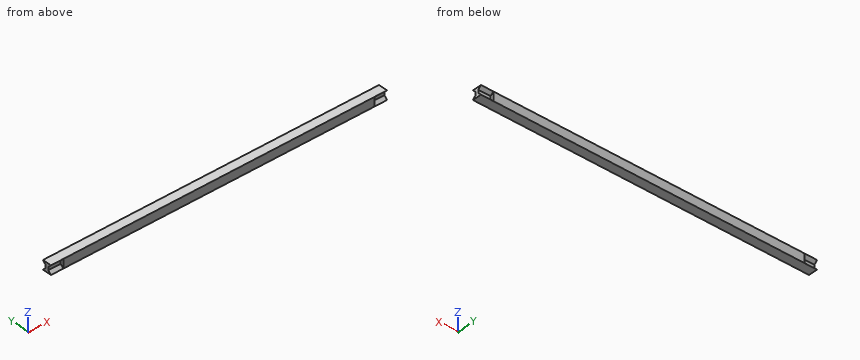
from build123d import *

# Parameters (mm, degrees)
SKICA1_W                = 202
SKICA1_H                = 5.9
P_IDAT_VYSUNUT_M1_DEPTH = 5.9
P_IDAT_VYSUNUT_M2_DEPTH = 8
P_IDAT_VYSUNUT_M3_DEPTH = 8


with BuildPart() as part:
    # Skica1 → Přidat vysunutím1 (new body)
    with BuildSketch(Plane(origin=(0, 0, 0), x_dir=(1, 0, 0), z_dir=(0, 1, 0))):
        with Locations((101, 2.95)):
            Rectangle(SKICA1_W, SKICA1_H)
    extrude(amount=P_IDAT_VYSUNUT_M1_DEPTH)

    # Skica2 → Přidat vysunutím2 (add)
    with BuildSketch(Plane.ZY):
        Polygon((-5.9, 5.9), (-5.9, 0), (-4, 1.9), (-1.9, 1.9), (0, 0), (0, 5.9), (-1.9, 4), (-4, 4), align=None)
    extrude(amount=P_IDAT_VYSUNUT_M2_DEPTH)

    # Skica3 → Přidat vysunutím3 (add)
    with BuildSketch(Plane(origin=(202, 0, 0), x_dir=(0, 0, -1), z_dir=(1, 0, 0))):
        Polygon((0, 5.9), (0, 0), (1.9, 1.9), (4, 1.9), (5.9, 0), (5.9, 5.9), (4, 4), (1.9, 4), align=None)
    extrude(amount=P_IDAT_VYSUNUT_M3_DEPTH)


solid = part.part
Verification items for the finished model (mm, model axes). Round coordinates to 2 decimals unless told otherwise and drop trailing zeros. Loops run counter-clockwise (first coordinate to the right, second up) from the corner with the lowest first, then second, coordinate; pieces in that order, holes last. Notation, with made-up numbers: (64, 76.5) - (120, 76.5) arc R20 ccw to (120, 113.5) - close; hole circle Ø3 at (61.5, -23.75). An arc over 180 degrees is marked (long way). Answer in a Markdown table with one row per item. Add a question column.
Q1. Material ranges on line 1 (X direction, y = 5.65, z = -0.65), recorded low to high.
Q2. Section check A-A on y = 4.95. Enter the section's corners in (x, z).
Q3. Gauge pin test, flat ends, axial feed: pin 1 (0.6 mm diameter, centred on y = 0.5, z = -4, fed in from +X); pin 2 (1 mm diameter, centred on x = 206, z = -3, fed in from -Y); pin 3 (0.6 mm diameter, centred on y = 5.5, z = -4, fed in from -X). Record the tip position at first contact, or that the pin passes through.
Found:
| question | item | result |
|---|---|---|
| 1 | line 1 | x = 0 to 202 |
| 2 | outline | (-8, -5.9) - (210, -5.9) - (210, -4.95) - (202, -4.95) - (202, -0.95) - (210, -0.95) - (210, 0) - (-8, 0) - (-8, -0.95) - (0, -0.95) - (0, -4.95) - (-8, -4.95) - close |
| 3 | pin 1 | stops at x = 202 |
| 3 | pin 2 | stops at y = 1.9 |
| 3 | pin 3 | stops at x = 0 |
